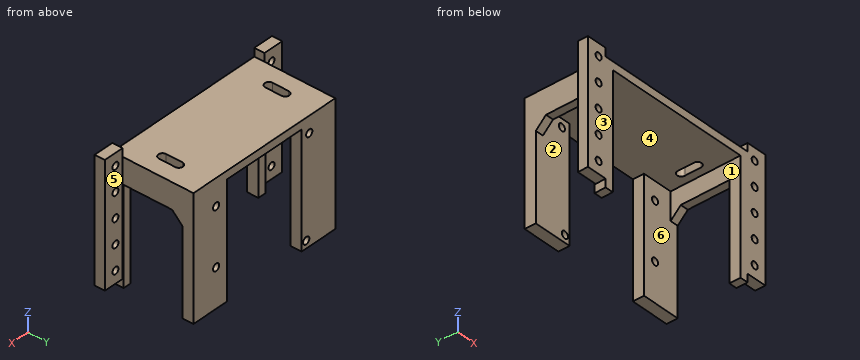
```python
from build123d import *

# Parameters (mm, degrees)
SKETCH_1_W          = 80
SKETCH_1_H          = 60
EXTRUDE_1_DEPTH     = 20
SKETCH_2_W          = 72
SKETCH_2_H          = 56
CUT_EXTRUDE_1_DEPTH = 70
SKETCH_3_W          = 47.385697094
SKETCH_3_H          = 29
CUT_EXTRUDE_2_DEPTH = 80
SKETCH_4_W          = 10
SKETCH_4_H          = 60
EXTRUDE_2_DEPTH     = 5
SKETCH_5_R          = 1.7
CUT_EXTRUDE_3_DEPTH = 25
SKETCH_6_W          = 15
SKETCH_6_H          = 56
EXTRUDE_3_DEPTH     = 5.5
SKETCH_8_R          = 1.75
CUT_EXTRUDE_5_DEPTH = 10
CHAMFER_1_SIZE      = 5
CUT_EXTRUDE_8_DEPTH = 10


with BuildPart() as part:
    # 草图1 → 凸台-拉伸1 (new, symmetric)
    with BuildSketch(Plane(origin=(0, 0, 0), x_dir=(1, 0, 0), z_dir=(0, 1, 0))):
        Rectangle(SKETCH_1_W, SKETCH_1_H)
    extrude(amount=EXTRUDE_1_DEPTH, both=True)

    # 草图2 → 切除-拉伸1 (cut)
    with BuildSketch(Plane(origin=(0, 20, 0), x_dir=(1, 0, 0), z_dir=(0, 1, 0))):
        with Locations((0, 2)):
            Rectangle(SKETCH_2_W, SKETCH_2_H)
    extrude(amount=-CUT_EXTRUDE_1_DEPTH, mode=Mode.SUBTRACT)

    # 草图3 → 切除-拉伸2 (cut)
    with BuildSketch(Plane(origin=(40, 0, 0), x_dir=(0, 0, -1), z_dir=(1, 0, 0))):
        with Locations((6.307151453, 0)):
            Rectangle(SKETCH_3_W, SKETCH_3_H)
    extrude(amount=-CUT_EXTRUDE_2_DEPTH, mode=Mode.SUBTRACT)

    # 草图4 → 凸台-拉伸2 (add)
    with BuildSketch(Plane.XZ.offset(20)):
        with Locations((-45, 4)):
            Rectangle(SKETCH_4_W, SKETCH_4_H)
        with Locations((45, 4)):
            Rectangle(SKETCH_4_W, SKETCH_4_H)
    extrude(amount=-EXTRUDE_2_DEPTH)

    # 草图5 → 切除-拉伸3 (cut)
    with BuildSketch(Plane(origin=(0, -15, 0), x_dir=(1, 0, 0), z_dir=(0, 1, 0))):
        with Locations(Location((-44, 20, 0), (0, 0, 270))):
            Circle(SKETCH_5_R)
        with Locations(Location((-44, 8, 0), (0, 0, 270))):
            Circle(SKETCH_5_R)
        with Locations(Location((-44, -4, 0), (0, 0, 270))):
            Circle(SKETCH_5_R)
        with Locations(Location((-44, -16, 0), (0, 0, 270))):
            Circle(SKETCH_5_R)
        with Locations(Location((-44, -28, 0), (0, 0, 270))):
            Circle(SKETCH_5_R)
        with Locations(Location((44, -28, 0), (0, 0, 90))):
            Circle(SKETCH_5_R)
        with Locations(Location((44, -16, 0), (0, 0, 90))):
            Circle(SKETCH_5_R)
        with Locations(Location((44, -4, 0), (0, 0, 90))):
            Circle(SKETCH_5_R)
        with Locations(Location((44, 8, 0), (0, 0, 90))):
            Circle(SKETCH_5_R)
        with Locations(Location((44, 20, 0), (0, 0, 90))):
            Circle(SKETCH_5_R)
    extrude(amount=-CUT_EXTRUDE_3_DEPTH, mode=Mode.SUBTRACT)

    # 草图6 → 凸台-拉伸3 (add)
    with BuildSketch(Plane(origin=(0, 20, 0), x_dir=(1, 0, 0), z_dir=(0, 1, 0))):
        with Locations((-28.5, 2)):
            Rectangle(SKETCH_6_W, SKETCH_6_H)
        with Locations((28.5, 2)):
            Rectangle(SKETCH_6_W, SKETCH_6_H)
    extrude(amount=-EXTRUDE_3_DEPTH)

    # 草图8 → 切除-拉伸5 (cut)
    with BuildSketch(Plane(origin=(0, 20, 0), x_dir=(1, 0, 0), z_dir=(0, 1, 0))):
        with Locations(Location((-25.32, -22, 0), (0, 0, 270))):
            Circle(SKETCH_8_R)
        with Locations(Location((-23.61, 26.395, 0), (0, 0, 270))):
            Circle(SKETCH_8_R)
        with Locations(Location((27.2, 10.96, 0), (0, 0, 270))):
            Circle(SKETCH_8_R)
        with Locations(Location((27.2, -17, 0), (0, 0, 270))):
            Circle(SKETCH_8_R)
    extrude(amount=-CUT_EXTRUDE_5_DEPTH, mode=Mode.SUBTRACT)

    # 倒角1
    chamfer_1_edges = [part.edges().sort_by_distance(p)[0] for p in [
        (38, 14.5, 17.385697094),
        (-38, 14.5, 17.385697094),
    ]]
    chamfer(chamfer_1_edges, length=CHAMFER_1_SIZE)

    # 草图10 → 切除-拉伸8 (cut)
    with BuildSketch(Plane.XY.offset(30)):
        with BuildLine():
            Line((-28, 4), (-28, -4))
            ThreePointArc((-28, -4), (-30, -6), (-32, -4))
            Line((-32, -4), (-32, 4))
            ThreePointArc((-32, 4), (-30, 6), (-28, 4))
        make_face()
        with BuildLine():
            Line((28, 4), (28, -4))
            ThreePointArc((28, -4), (30, -6), (32, -4))
            Line((32, -4), (32, 4))
            ThreePointArc((32, 4), (30, 6), (28, 4))
        make_face()
    extrude(amount=-CUT_EXTRUDE_8_DEPTH, mode=Mode.SUBTRACT)


solid = part.part
```
Model file for the job. Use its own axes, mm. Face numbers are marked on the shaded views. A direction names the side the tool comes from. Give positions to 0.01 mm unless a question says otherwise; leave off trailing zeros. Loops run counter-clockwise (first coordinate to the right, second up) from the corner with the lowest first, then second, coordinate; pieces in that order, holes last. Notation, with made-up numbers: (60, -39) -> (108, -39) arc R17 ccw to (108, -15) -> close; hole circle Ø11 at (75.5, 13.5). An arc over 180 degrees is marked (long way). Use CSV: the item, a comma, the result in double quotes. Start each with the question number.
1) Slice it at A-A on z = 28. Give the cut face in (x, y), plus the area to 3 significant figures.
2) Tool access for the marked faces 4, 5 and 6: list every direction of +Z, -Z, +X, -X, +Y, -Y with a clear straight run to the whole face (end or side of a thin tool).
3) Flat gauge pins, fed straight in: pin 1 Ø4 at (x, y) = (-43, -18) entering from -Z; pin 2 Ø12 at (x, y) = (14.5, -11.5) entering from -Z; pin 3 Ø3 at (y, z) = (-1.5, 27.5) entering from -X. Where does each tip first touch, or does it go through?
4) Slice it at D-D on z = -8. Give the cut face in (x, y), plus the area to 3 significant figures.
5) Slice it at B-B on x = 44. Give the cut face in (y, z), plus the area to 3 significant figures.
6) Mould opens along Y. For the marked faces 1, 2 and 3 say: released by +Y, released by -Y, zero draft, split by the parting line, or undercut.
7) Wall check: line 1 (Z direction, x = 44, y = -17); line 2 (Z direction, x = 27, y = 16); line 3 (X direction, y = -17.6, z = -8). Give the ranges that are in metal, low to high.
8) Slice it at C-C on x = -30. Give the cut face in (y, z), plus the area to 3 significant figures.
Computed values:
1,outline,"(-50, -20) -> (-45.7, -20) -> (-45.7, -15) -> (-50, -15) -> close; (-42.3, -20) -> (42.3, -20) -> (42.3, -15) -> (40, -15) -> (40, 20) -> (-40, 20) -> (-40, -15) -> (-42.3, -15) -> close; (45.7, -20) -> (50, -20) -> (50, -15) -> (45.7, -15) -> close; hole (-32, -4) arc R2 ccw to (-28, -4) -> (-28, 4) arc R2 ccw to (-32, 4) -> close; hole (28, -4) arc R2 ccw to (32, -4) -> (32, 4) arc R2 ccw to (28, 4) -> close"
1,area,"3,180 mm^2"
2,face 4,"-Z, -Y"
2,face 5,"+Z, -Z, +X, +Y"
2,face 6,"-Z"
3,pin 1,"stops at z = -26"
3,pin 2,"stops at z = 26"
3,pin 3,"stops at x = -40"
4,outline,"(-50, -20) -> (-45.7, -20) -> (-45.7, -15) -> (-50, -15) -> close; (-42.3, -20) -> (-36, -20) -> (-36, -14.5) -> (-40, -14.5) -> (-40, -15) -> (-42.3, -15) -> close; (-40, 14.5) -> (-21, 14.5) -> (-21, 20) -> (-40, 20) -> close; (21, 14.5) -> (40, 14.5) -> (40, 20) -> (21, 20) -> close; (36, -20) -> (42.3, -20) -> (42.3, -15) -> (40, -15) -> (40, -14.5) -> (36, -14.5) -> close; (45.7, -20) -> (50, -20) -> (50, -15) -> (45.7, -15) -> close"
4,area,"319 mm^2"
5,outline,"(-20, -26) -> (-15, -26) -> (-15, -21.7) -> (-20, -21.7) -> close; (-20, -18.3) -> (-15, -18.3) -> (-15, -9.7) -> (-20, -9.7) -> close; (-20, -6.3) -> (-15, -6.3) -> (-15, 2.3) -> (-20, 2.3) -> close; (-20, 5.7) -> (-15, 5.7) -> (-15, 14.3) -> (-20, 14.3) -> close; (-20, 17.7) -> (-15, 17.7) -> (-15, 26.3) -> (-20, 26.3) -> close; (-20, 29.7) -> (-15, 29.7) -> (-15, 34) -> (-20, 34) -> close"
5,area,"215 mm^2"
6,face 1,"zero draft"
6,face 2,"undercut"
6,face 3,"released by -Y"
7,line 1,"z = -26 to -21.7, -18.3 to -9.7, -6.3 to 2.3, 5.7 to 14.3, 17.7 to 26.3, 29.7 to 34"
7,line 2,"z = -30 to -12.7, -9.22 to 15.26, 18.74 to 30"
7,line 3,"x = -50 to -45.7, -42.3 to -36, 36 to 42.3, 45.7 to 50"
8,outline,"(-20, 26) -> (-6, 26) -> (-6, 30) -> (-20, 30) -> close; (6, 26) -> (14.5, 26) -> (14.5, -30) -> (20, -30) -> (20, 30) -> (6, 30) -> close"
8,area,"420 mm^2"
